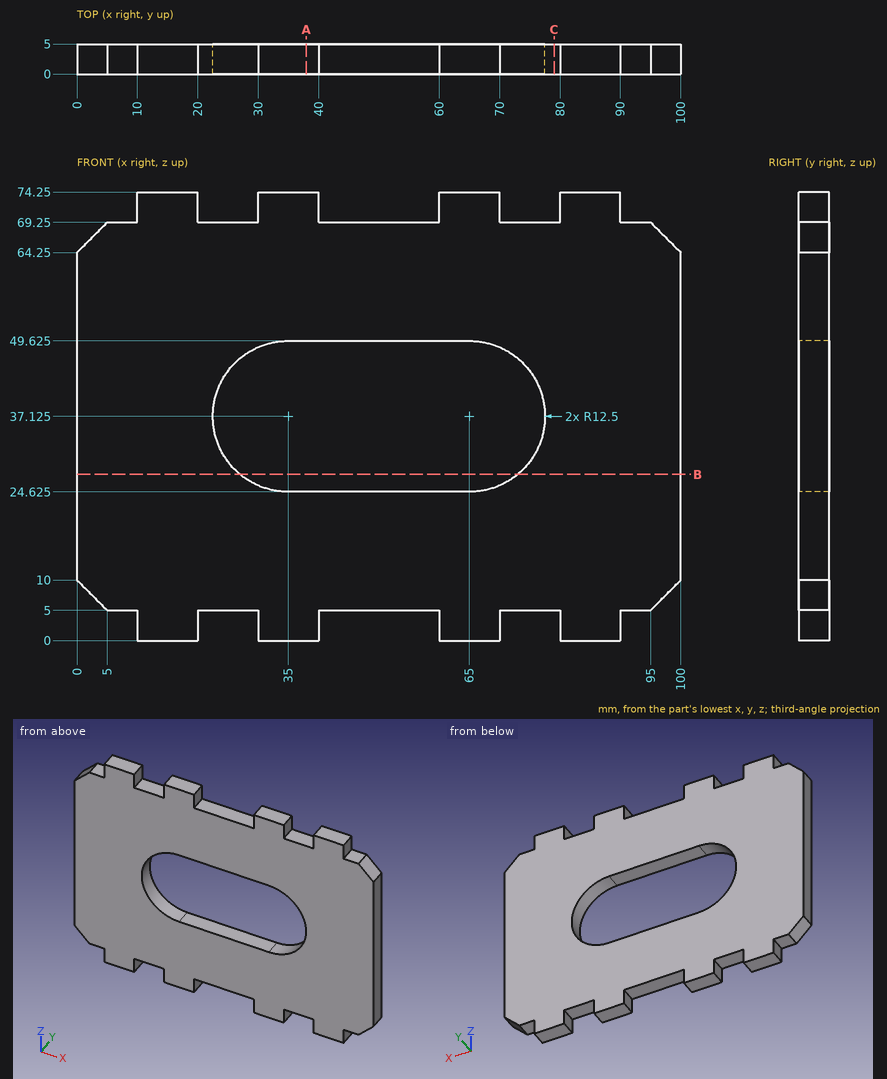
Verification items for this drawing (mm, ordinates from the low corner). Give positions to 0.01 mm unless a question says otherwise; leave off trailing zeros. Write each loop counter-clockwise with the first axis right and the second up, starting at its lowest first coordinate (ties: lowest second). Pieces come first, ordered by that corner, then holes. Notation, with made-up numbers: (64.5, -34) -> (69.5, -34) arc R13 cw to (69.5, -12) -> close; hole circle Ø7 at (56.5, -30). An arc over 180 degrees is marked (long way). Use CSV: the item, a comma, the result in double quotes. Start each with the question number.
Q1. Depth check by flat-ended pin: P1, Ø1.5, axis at x = 7, y = 3.5, coming from the +Z side; P2, Ø2, axis at x = 74.5, z = 16, coming from the -Y side; P3, Ø1.5, axis at y = 2, z = 1.5, coming from the +X side; P4, Ø2.5, axis at y = 2, z = 72, coming from the -X side. Enter the tip coordinate at first touch or a pass-through.
Q2. Scan lines: line 1 along X through (y, z) = (3.7, 71.5); line 2 along Z through (x, y) = (41, 4.15) (3 decimals); line 3 along Z through (x, y) = (64.5, 3.4) (3 decimals). Record each from-to range of solid material in increasing order.
Q3. Cross-section at B-B on z = 27.5. Enter the section's corners in (x, y), and give its area (3 significant figures).
Q4. Cross-section at A-A on x = 38. Enter the section's corners in (y, z) (3 decimals), and give its area (3 significant figures).
Q5. Cross-section at C-C on x = 79. Enter the section's corners in (y, z).
Working result:
1,P1,"stops at z = 69.25"
1,P2,"stops at y = 0"
1,P3,"stops at x = 90"
1,P4,"stops at x = 10"
2,line 1,"x = 10 to 20, 30 to 40, 60 to 70, 80 to 90"
2,line 2,"z = 5 to 24.625, 49.625 to 69.25"
2,line 3,"z = 0 to 24.625, 49.625 to 74.25"
3,outline,"(0, 0) -> (27.02, 0) -> (27.02, 5) -> (0, 5) -> close; (72.98, 0) -> (100, 0) -> (100, 5) -> (72.98, 5) -> close"
3,area,"270 mm^2"
4,outline,"(0, 0) -> (5, 0) -> (5, 24.625) -> (0, 24.625) -> close; (0, 49.625) -> (5, 49.625) -> (5, 74.25) -> (0, 74.25) -> close"
4,area,"246 mm^2"
5,outline,"(0, 5) -> (5, 5) -> (5, 69.25) -> (0, 69.25) -> close"
